from build123d import *

# Parameters (mm, degrees)
ESTRUSIONE_ESTRUSIONE1_DEPTH = 2.5
SCHIZZO2_W                   = 15
SCHIZZO2_H                   = 23.5
ESTRUSIONE_ESTRUSIONE2_DEPTH = 23.5
SCHIZZO3_W                   = 17.5
SCHIZZO3_H                   = 23.5
ESTRUSIONE_ESTRUSIONE3_DEPTH = 4.5
SCHIZZO4_W                   = 17.5
SCHIZZO4_H                   = 28
ESTRUSIONE_ESTRUSIONE4_DEPTH = 4.5
SCHIZZO5_W                   = 15
SCHIZZO5_H                   = 23.5
TAGLIO_ESTRUSIONE1_DEPTH     = 23.5
ESTRUSIONE_ESTRUSIONE5_DEPTH = 2.5
SCHIZZO7_W                   = 8
SCHIZZO7_H                   = 2
ESTRUSIONE_ESTRUSIONE6_DEPTH = 1
SCHIZZO8_W                   = 8
SCHIZZO8_H                   = 2
ESTRUSIONE_ESTRUSIONE7_DEPTH = 1
SCHIZZO9_W                   = 8
SCHIZZO9_H                   = 2
ESTRUSIONE_ESTRUSIONE8_DEPTH = 1
SCHIZZO10_W                  = 8
SCHIZZO10_H                  = 2
ESTRUSIONE_ESTRUSIONE9_DEPTH = 1
FORO_6_3_6_3_1_D             = 6.3
FORO_6_3_6_3_1_DEPTH         = 5.5
FORO_6_3_6_3_2_D             = 6.3
FORO_6_3_6_3_2_DEPTH         = 5.5
RACCORDO1_R                  = 0.3
RACCORDO2_START              = -11
RACCORDO2_DEPTH              = 22
FORO_FILETTATO_M5_1_D        = 4.2


with BuildPart() as part:
    # Schizzo1 → Estrusione-Estrusione1 (new body)
    with BuildSketch(Plane(origin=(-10, 0, 0), x_dir=(0, -1, 0), z_dir=(-1, 0, 0))):
        with BuildLine():
            Line((-27.707106781, 4.792893219), (-28, 4.5))
            Line((-28, 4.5), (-4.5, 4.5))
            Line((-4.5, 4.5), (-4.5, 28))
            Line((-4.5, 28), (-4.792893219, 27.707106781))
            add(Edge.make_bspline(
                [(-4.792893219, 27.707106781), (-12.430964406, 20.069035594), (-20.069035594, 12.430964406), (-27.707106781, 4.792893219)],
                knots=[0, 0, 0, 0, 1, 1, 1, 1], degree=3))
        make_face()
    extrude(amount=-ESTRUSIONE_ESTRUSIONE1_DEPTH)

    # Schizzo2 → Estrusione-Estrusione2 (add)
    with BuildSketch(Plane(origin=(0, 0, 4.5), x_dir=(-1, 0, 0), z_dir=(0, 0, -1))):
        with Locations((0, 16.25)):
            Rectangle(SCHIZZO2_W, SCHIZZO2_H)
    extrude(amount=-ESTRUSIONE_ESTRUSIONE2_DEPTH)

    # Schizzo3 → Estrusione-Estrusione3 (add)
    with BuildSketch(Plane(origin=(0, 0, 4.5), x_dir=(-1, 0, 0), z_dir=(0, 0, -1))):
        with Locations((1.25, 16.25)):
            Rectangle(SCHIZZO3_W, SCHIZZO3_H)
    extrude(amount=ESTRUSIONE_ESTRUSIONE3_DEPTH)

    # Schizzo4 → Estrusione-Estrusione4 (add)
    with BuildSketch(Plane.XZ.offset(-4.5)):
        with Locations((-1.25, 14)):
            Rectangle(SCHIZZO4_W, SCHIZZO4_H)
    extrude(amount=ESTRUSIONE_ESTRUSIONE4_DEPTH)

    # Schizzo5 → Taglio-Estrusione1 (cut)
    with BuildSketch(Plane(origin=(0, 28, 0), x_dir=(-1, 0, 0), z_dir=(0, 1, 0))):
        with Locations((0, 16.25)):
            Rectangle(SCHIZZO5_W, SCHIZZO5_H)
    extrude(amount=-TAGLIO_ESTRUSIONE1_DEPTH, mode=Mode.SUBTRACT)

    # Schizzo6 → Estrusione-Estrusione5 (add)
    with BuildSketch(Plane(origin=(7.5, 0, 0), x_dir=(0, 0, -1), z_dir=(1, 0, 0))):
        with BuildLine():
            Line((-28, 0), (-28, 4.5))
            Line((-28, 4.5), (-27.707106492, 4.792893508))
            add(Edge.make_bspline(
                [(-4.792893219, 27.707106781), (-12.43096431, 20.06903569), (-20.069035401, 12.430964599), (-27.707106492, 4.792893508)],
                knots=[0, 0, 0, 0, 1, 1, 1, 1], degree=3))
            Line((-4.792893219, 27.707106781), (-4.5, 28))
            Line((-4.5, 28), (0, 28))
            Line((0, 28), (0, 0))
            Line((0, 0), (-28, 0))
        make_face()
    extrude(amount=ESTRUSIONE_ESTRUSIONE5_DEPTH)

    # Schizzo7 → Estrusione-Estrusione6 (add)
    with BuildSketch(Plane(origin=(0, 0, 0), x_dir=(-1, 0, 0), z_dir=(0, 0, -1))):
        with Locations((0, 5)):
            Rectangle(SCHIZZO7_W, SCHIZZO7_H)
    extrude(amount=ESTRUSIONE_ESTRUSIONE6_DEPTH)

    # Schizzo8 → Estrusione-Estrusione7 (add)
    with BuildSketch(Plane(origin=(0, 0, 0), x_dir=(-1, 0, 0), z_dir=(0, 0, -1))):
        with Locations((0, 24.5)):
            Rectangle(SCHIZZO8_W, SCHIZZO8_H)
    extrude(amount=ESTRUSIONE_ESTRUSIONE7_DEPTH)

    # Schizzo9 → Estrusione-Estrusione8 (add)
    with BuildSketch(Plane.XZ):
        with Locations((0, 24.5)):
            Rectangle(SCHIZZO9_W, SCHIZZO9_H)
    extrude(amount=ESTRUSIONE_ESTRUSIONE8_DEPTH)

    # Schizzo10 → Estrusione-Estrusione9 (add)
    with BuildSketch(Plane.XZ):
        with Locations((0, 5)):
            Rectangle(SCHIZZO10_W, SCHIZZO10_H)
    extrude(amount=ESTRUSIONE_ESTRUSIONE9_DEPTH)

    # Foro Ø6.3 (6.3)-1
    with Locations(Plane(origin=(0, 4.5, 0), x_dir=(1, 0, 0), z_dir=(0, 1, 0))):
        with Locations((0, -20)):
            Hole(FORO_6_3_6_3_1_D / 2, depth=FORO_6_3_6_3_1_DEPTH)

    # Foro Ø6.3 (6.3)-2
    with Locations(Plane.XY.offset(4.5)):
        with Locations((0, 20)):
            Hole(FORO_6_3_6_3_2_D / 2, depth=FORO_6_3_6_3_2_DEPTH)

    # Raccordo1
    raccordo1_edges = [part.edges().sort_by_distance(p)[0] for p in [
        (-4, 23.5, -0.5),
        (-4, 25.5, -0.5),
        (4, 25.5, -0.5),
        (4, 23.5, -0.5),
        (4, -0.5, 25.5),
        (-4, -0.5, 25.5),
        (-4, -0.5, 23.5),
        (4, -0.5, 23.5),
        (4, -0.5, 6),
        (-4, -0.5, 6),
        (-4, -0.5, 4),
        (4, -0.5, 4),
        (-4, 4, -0.5),
        (-4, 6, -0.5),
        (4, 6, -0.5),
        (4, 4, -0.5),
    ]]
    fillet(raccordo1_edges, radius=RACCORDO1_R)

    # Raccordo2: read off the stored shape, not the designer's step
    # Raccordo2 outline → Raccordo2 (cut)
    with BuildSketch(Plane.YZ.offset(RACCORDO2_START)):
        with BuildLine():
            ThreePointArc((4.5, 27.910179721), (4.655566811, 27.82179701), (4.792893508, 27.707106492))
            Line((4.792893508, 27.707106492), (4.5, 28))
            Line((4.5, 28), (4.5, 27.910179721))
        make_face()
        with BuildLine():
            ThreePointArc((4.085786438, 28), (4.297706563, 27.97728699), (4.5, 27.910179721))
            Line((4.5, 27.910179721), (4.5, 28))
            Line((4.5, 28), (4.085786438, 28))
        make_face()
        with BuildLine():
            Line((28, 4.5), (27.707106781, 4.792893219))
            ThreePointArc((27.707106781, 4.792893219), (27.821797127, 4.655566644), (27.910179722, 4.5))
            Line((27.910179722, 4.5), (28, 4.5))
        make_face()
        with BuildLine():
            Line((28, 4.5), (27.910179722, 4.5))
            ThreePointArc((27.910179722, 4.5), (27.97728699, 4.297706563), (28, 4.085786438))
            Line((28, 4.085786438), (28, 4.5))
        make_face()
    extrude(amount=RACCORDO2_DEPTH, mode=Mode.SUBTRACT)

    # Foro filettato M5-1 (through all)
    with Locations(Plane(origin=(10, 12, 12), x_dir=(0, 0, 1), z_dir=(1, 0, 0))):
        with Locations((0, 0)):
            Hole(FORO_FILETTATO_M5_1_D / 2)


solid = part.part
Source: CAD feature listing. Evaluate the final solid. Frame: model axes, mm. A direction names the side the tool comes from. Give positions to 0.01 mm unless a question says otherwise; leave off trailing zeros. Loops run counter-clockwise (first coordinate to the right, second up) from the corner with the lowest first, then second, coordinate; pieces in that order, holes last. Notation, with made-up numbers: (-2.75, 66) -> (31.25, 66) arc R27 cw to (31.25, 104) -> close; hole circle Ø9 at (79, 43.25). An arc over 180 degrees is marked (long way). Use a Markdown table: item, result. Add a question column.
1) Reachability of faces 4 (the face through (0.1, 4, -0.5)), 5 (the face through (-4, -0.5, 5)), 6 (the face through (0, 16, 4.5)), 7 (the face through (4, -0.5, 5)) from +Z, -Z, +X, -X, +Y, -Y: full face, straight path, thin tool, end or side. Return the list, or none.
2) First-contact query: pin 1 (10 mm diameter, centred on x = 6, z = 11, fed in from -Y); pin 2 (1 mm diameter, centred on x = -3.5, z = 6.5, fed in from +Y); pin 3 (5 mm diameter, centred on x = 2.5, y = 12, fed in from -Z); pin 4 (10 mm diameter, centred on x = 4.5, y = 7.5, fed in from -Z). Flat tips, straight axial feed; report the tip coordinate or a pass-through.
3) Section query C-C, the plane x = 0. Count the separate pieces of the cut face and the enclosed holes in it, then the cut area to 3 significant figures.
4) Pull-direction query (Z, two-part tool) for faces 1 (the face through (-8.768, 9.918, 12.273)), 2 (the face through (-4, -0.5, 24.5)), 3 (the face through (-0.1, -0.5, 4)); classes: +Z half, -Z half, draft (parallel to the pull), parting line (faces both ways), or undercut.
5) Section query B-B, the plane y = 20. Return the cut outline in (x, z), then the cut area to 3 significant figures.
6) Section query A-A, the plane z = 12. Return the cut outline in (x, y).
7) Line query: line 1 along X through (y, z) = (21, 10.5); line 2 along Y through (x, z) = (0, 1.2); line 3 along Z through (x, y) = (5, 4.75). Output: solid intervals per line, ascending. Write a range as [from, to].
Numbers:
| question | item | result |
|---|---|---|
| 1 | face 4 | -Z, +X, -X, -Y |
| 1 | face 5 | +Z, -Z, -X, -Y |
| 1 | face 6 | +Z, +Y |
| 1 | face 7 | +Z, -Z, +X, -Y |
| 2 | pin 1 | stops at y = 0 |
| 2 | pin 2 | stops at y = 4.5 |
| 2 | pin 3 | stops at z = 0 |
| 2 | pin 4 | stops at z = -1 |
| 3 | separate pieces | 3 |
| 3 | enclosed holes | 0 |
| 3 | area | 183 mm2 |
| 4 | face 1 | undercut |
| 4 | face 2 | draft |
| 4 | face 3 | -Z half |
| 5 | outline | (-10, 0) -> (-3.15, 0) -> (-3.15, 4.5) -> (-7.5, 4.5) -> (-7.5, 12.5) -> (-10, 12.5) -> close; (3.15, 0) -> (10, 0) -> (10, 12.5) -> (7.5, 12.5) -> (7.5, 4.5) -> (3.15, 4.5) -> close |
| 5 | area | 102 mm2 |
| 6 | outline | (-10, 0) -> (10, 0) -> (10, 9.9) -> (7.5, 9.9) -> (7.5, 4.5) -> (-7.5, 4.5) -> (-7.5, 9.9) -> (-10, 9.9) -> close; (-10, 14.1) -> (-7.5, 14.1) -> (-7.5, 20.5) -> (-10, 20.5) -> close; (7.5, 14.1) -> (10, 14.1) -> (10, 20.5) -> (7.5, 20.5) -> close |
| 7 | line 1 | x = [-10, -7.5], [7.5, 10] |
| 7 | line 2 | y = [0, 16.85], [23.15, 28] |
| 7 | line 3 | z = [0, 4.5] |
